Autodesk Inventor part; units mm, degrees
ref_plane "YZ Plane" through (0, 0, 0) normal (1, 0, 0) x (0, 1, 0)
ref_plane "XZ Plane" through (0, 0, 0) normal (0, 1, 0) x (-1, 0, 0)
ref_plane "XY Plane" through (0, 0, 0) normal (0, 0, 1) x (1, 0, 0)
sketch "Sketch1" plane through (0, 0, 0) normal (0, 1, 0) x (-1, 0, 0)
  circle A0 centre (0, 0) radius 12.5
  dimension "d0" = 25
extrude "Extrusion1" add sketch "Sketch1" along normal blind 2.5
sketch "Sketch2" plane through (0, 2.5, 0) normal (0, 1, 0) x (1, 0, 0)
  circle A0 centre (0, 0) radius 11.5
  dimension "d3" = 23
extrude "Extrusion2" cut sketch "Sketch2" against normal blind 1
sketch "Sketch3" plane through (0, 2.5, 0) normal (0, 1, 0) x (1, 0, 0)
  circle A0 centre (0, 0) radius 11.5
  circle A1 centre (0, 0) radius 12.5
  line L0 (-8.2614, -8) -> (-9.6047, -8)
  line L1 (-8.2614, 8) -> (-9.6047, 8)
extrude "Extrusion3" cut sketch "Sketch3" against normal up to surface (1 mm away) contours A0 L0 A1 L1 picked at (-11.7871, 0)
sketch "Sketch6" plane through (0, 2.5, 0) normal (0, 1, 0) x (1, 0, 0)
  arc A0 (-9.6047, -8) -> (-9.6047, 8) centre (0, 0) ccw
  arc A1 (-8.2614, -8) -> (-8.2614, 8) centre (0, 0) ccw
  line L0 (-9.6047, 8) -> (-8.2614, 8)
  line L1 (-8.2614, -8) -> (-9.6047, -8)
extrude "Extrusion5" add sketch "Sketch6" along normal blind 1
sketch "Sketch7" plane through (0, 3.5, 0) normal (0, 1, 0) x (1, 0, 0)
  arc A0 (-8.2614, -8) -> (-8.2614, 8) centre (0, 0) ccw
  line L0 (-9.6047, 8) -> (-8.2614, 8)
  line L1 (-8.2614, -8) -> (-9.6047, -8)
  arc A1 (-9.6047, -8) -> (-9.6047, 8) centre (0, 0) ccw
extrude "Extrusion6" add sketch "Sketch7" along normal blind 5
sketch "Sketch8" plane through (0, 0, 0) normal (0, -1, 0) x (1, 0, 0)
  circle A0 centre (0, 0) radius 12.5
extrude "Extrusion7" add sketch "Sketch8" along normal blind 4.5
sketch "Sketch9" plane through (0, -4.5, 0) normal (0, -1, 0) x (1, 0, 0)
  circle A0 centre (0, 0) radius 12.5
extrude "Extrusion8" add sketch "Sketch9" along normal blind 5
properties part number "Heis_kopp" material "S355J2+N"
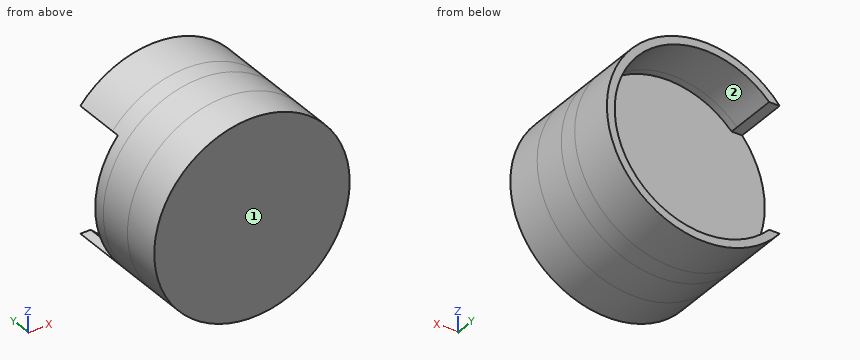
Part model, mm, in its own coordinate system. Face numbers are marked on the shaded views. Coordinates: 2 decimals unless noted, no trailing zeros. Order: outer loops, then holes, each group sorted by start corner. A loop starts at its lowest first (then second) coordinate and runs counter-clockwise, first axis right, second up. Notation, with made-up numbers: (51, 64.5) -> (103, 64.5) arc R27 ccw to (103, 87.5) -> close; hole circle Ø6 at (87, 76). An arc over 180 degrees is marked (long way). Put each result on its own line as item: value. Start each with the question number.
(1) Band-saw the part on C-C (y = 4.5). Give the cut face in (x, z), then the cut area to 3 significant figures.
(2) Band-saw the part on A-A (z = 0). Give the cut face in (x, y).
(3) Band-saw the part on D-D (z = -6.5). Give the cut face in (x, y).
(4) Mould opens along Z. For the marked faces 1 and 2 say: pulls with the +Z half, pulls with the -Z half, needs draft (parallel to the pull), parting line crosses it, or undercut.
(5) Probe line 1 along Z through (x, y) = (0, 2.35); line 2 along Y through (x, z) = (1.75, -8.25); line 3 along Z through (x, y) = (-8.75, 2.75). List the from-to ranges inside material, lowest first. Write a range as [from, to].
(6) Pin check, flat tips, straight feed: pin 1 Ø1.1 at (x, y) = (-9, 5.5) entering from +Z; pin 2 Ø4 at (x, y) = (4, -1) entering from -Z; pin 3 Ø6 at (x, y) = (4.5, 4.5) entering from -Z. Stop position of each tip, or through.
(7) Band-saw the part on B-B (x = 0). Give the cut face in (y, z).
Determined:
1. outline: (-9.6, -8) arc R12.5 ccw (long way) to (-9.6, 8) -> (-8.26, 8) arc R11.5 cw (long way) to (-8.26, -8) -> close
1. area: 57.9 mm²
2. outline: (-12.5, -9.5) -> (12.5, -9.5) -> (12.5, 8.5) -> (11.5, 8.5) -> (11.5, 1.5) -> (-12.5, 1.5) -> close
3. outline: (-10.68, -9.5) -> (10.68, -9.5) -> (10.68, 8.5) -> (9.49, 8.5) -> (9.49, 1.5) -> (-10.68, 1.5) -> close
4. face 1: needs draft
4. face 2: undercut
5. line 1: z = [-12.5, -11.5], [11.5, 12.5]
5. line 2: y = [-9.5, 1.5]
5. line 3: z = [-8.93, -8], [8, 8.93]
6. pin 1: stops at z = 9.21
6. pin 2: stops at z = -12.34
6. pin 3: stops at z = -12.41
7. outline: (-9.5, -12.5) -> (8.5, -12.5) -> (8.5, -11.5) -> (1.5, -11.5) -> (1.5, 11.5) -> (8.5, 11.5) -> (8.5, 12.5) -> (-9.5, 12.5) -> close
